The drawing under review shows one solid part. Ordinate dimensions are in mm from its lowest x, y, z. Give positions to 0.01 mm unless a question says otherwise; leave off trailing zeros. Order: outer loops, then holes, each group sorted by start corner. A loop starts at its lowest first (then second) coordinate and runs counter-clockwise, first axis right, second up. Notation, with made-up numbers: (-25, 69) - (3, 69) arc R21 cw to (3, 76) - close; hole circle Ø11 at (5.25, 62.5). An arc over 180 degrees is marked (long way). Write item = value, one per line. Start each with the question number.
1. We need section B-B, the plane y = 14. Give the boundary of the cut face in (x, z), and give its area (3 significant figures).
2. Wall thickness on probe 1 along Y at (x, z) = (19.78, 8.25); probe 2 along Z at (x, y) = (11, 34); probe 3 along X at (y, z) = (6, 6.5): over which ranges is each line inside the solid? List them lowest first.
3. Mouldability with a two-part tool opening along X and no side actions: class the marked faces 1, 2, 3 and 4 as pulls with the +X half, pulls with the -X half, needs draft (parallel to the pull), parting line crosses it, or undercut.
4. For P1, Ø3.5, axis at y = 35, z = 2, coming from the -X side; P2, Ø2.5, axis at x = 2, z = 1.5, coming from the +Y side; P3, Ø3.5, axis at x = 38, z = 1, coming from the -Y side; P4, Ø6, axis at y = 17.5, z = 3, coming from the -X side, all flat-tipped, find the tip position at first contact; note any pin that passes through.
5. We need section A-A, the plane x = 19.78. Give the boundary of the cut face in (y, z), and give its area (3 significant figures).
6. We need section C-C, the plane z = 4. Give the boundary of the cut face in (x, y), and give its area (3 significant figures).
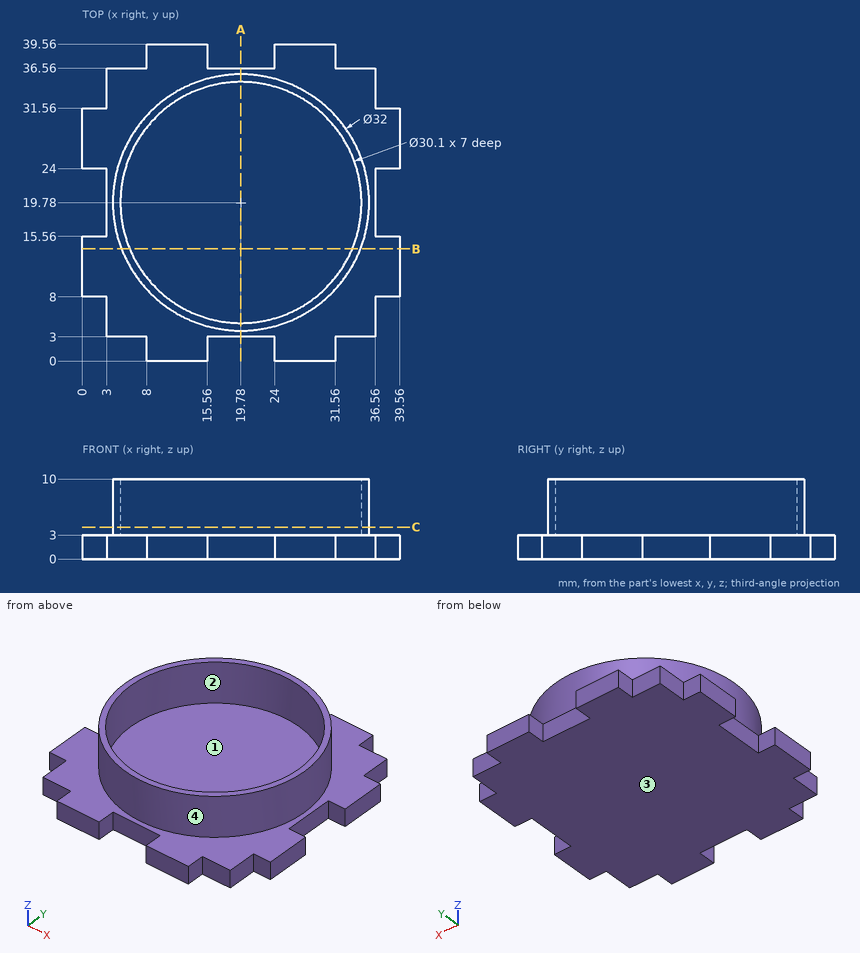
Model answer:
q1.outline = (0, 0) - (39.56, 0) - (39.56, 3) - (34.7, 3) - (34.7, 10) - (33.68, 10) - (33.68, 3) - (5.88, 3) - (5.88, 10) - (4.86, 10) - (4.86, 3) - (0, 3) - close
q1.area = 133 mm2
q2.probe_1 = 3.78 to 4.73, 34.83 to 35.78
q2.probe_2 = 0 to 3
q2.probe_3 = 11.65 to 13.73, 25.83 to 27.91
q3.face_1 = undercut
q3.face_2 = undercut
q3.face_3 = needs draft
q3.face_4 = parting line crosses it
q4.P1 = 3
q4.P2 = 36.56
q4.P3 = 3
q4.P4 = 0
q5.outline = (3, 0) - (36.56, 0) - (36.56, 3) - (35.78, 3) - (35.78, 10) - (34.83, 10) - (34.83, 3) - (4.73, 3) - (4.73, 10) - (3.78, 10) - (3.78, 3) - (3, 3) - close
q5.area = 114 mm2
q6.outline = circle Ø32 at (19.78, 19.78); hole circle Ø30.1 at (19.78, 19.78)
q6.area = 92.7 mm2
